Design review of the part built by this model. Coordinates are the model's own, in mm. Give positions to 0.01 mm unless a question says otherwise; leave off trailing zeros.
```python
from build123d import *

# Parameters (mm, degrees)
SKETCH3_R          = 5
SKETCH6_R          = 5
SKETCH7_R          = 7.5
CUT_EXTRUDE1_DEPTH = 123.474487302


with BuildPart() as part:
    # Sketch1 → Loft1 section 0
    with BuildSketch(Plane(origin=(0, 0, 0), x_dir=(0, 0, -1), z_dir=(1, 0, 0))):
        with BuildLine():
            Line((40, 40), (-40, 40))
            Line((-40, 40), (-40, -40))
            Line((-40, -40), (40, -40))
            Line((40, -40), (40, 40))
        make_face()
    # Sketch2 → Loft1 section 1
    with BuildSketch(Plane(origin=(-100, 0, 0), x_dir=(0, 0, -1), z_dir=(1, 0, 0))):
        with BuildLine():
            Line((50, 50), (-50, 50))
            Line((-50, 50), (-50, -50))
            Line((-50, -50), (50, -50))
            Line((50, -50), (50, 50))
        make_face()
    loft()

    # Cut-Sweep2: sweep along a path in Sketch4
    with BuildLine(Plane(origin=(0, 0, 0), x_dir=(1, 0, 0), z_dir=(0, 1, 0))) as cut_sweep2_path:
        Line((0, 15), (-100, 25))
    # Sketch3 → Cut-Sweep2 (sweep, cut)
    with BuildSketch(Plane(origin=(0, 0, 0), x_dir=(0, 0, -1), z_dir=(1, 0, 0))):
        with Locations((15, 0)):
            Circle(SKETCH3_R)
    cut_sweep2 = sweep(path=cut_sweep2_path.line, mode=Mode.SUBTRACT)

    # Cut-Sweep3: sweep along a path in Sketch5
    with BuildLine(Plane.XY) as cut_sweep3_path:
        Line((0, 15), (-100, 25))
    # Sketch6 → Cut-Sweep3 (sweep, cut)
    with BuildSketch(Plane(origin=(0, 0, 0), x_dir=(0, 0, -1), z_dir=(1, 0, 0))):
        with Locations((0, 15)):
            Circle(SKETCH6_R)
    cut_sweep3 = sweep(path=cut_sweep3_path.line, mode=Mode.SUBTRACT)

    # Mirror1: Cut-Sweep2 across plane
    add(cut_sweep2.mirror(Plane.XY), mode=Mode.SUBTRACT)

    # Mirror2: Cut-Sweep3 across plane
    add(cut_sweep3.mirror(Plane.ZX), mode=Mode.SUBTRACT)

    # Sketch7 → Cut-Extrude1 (cut, through all)
    with BuildSketch(Plane(origin=(0, 0, 0), x_dir=(0, 0, -1), z_dir=(1, 0, 0))):
        Circle(SKETCH7_R)
    extrude(amount=-CUT_EXTRUDE1_DEPTH, mode=Mode.SUBTRACT)


solid = part.part
```
1. Draft analysis for pull direction Z (two halves, no side actions). For faces 1 (the face through (-49.3, 0.33, 7.493)), 2 (the face through (-100, 13, 11)), state which applies: pulls with the +Z half, pulls with the -Z half, needs draft (parallel to the pull), parting line crosses it, or undercut.
Recorded:
face 1: undercut
face 2: needs draft
2. For line 1 along Y through (x, z) = (-68, 4.5); line 2 along Z through (x, y) = (-31.5, -1); line 3 along Y through (x, z) = (-47, 0), list the stretches that pass through material, from the lowest coordinate up.
Recorded:
line 1: y = -46.8 to -23.98, -19.62 to -6, 6 to 19.62, 23.98 to 46.8
line 2: z = -43.15 to -23.05, -13.25 to -7.43, 7.43 to 13.25, 23.05 to 43.15
line 3: y = -44.7 to -24.7, -14.7 to -7.5, 7.5 to 14.7, 24.7 to 44.7
3. For pin 1 (1.5 mm diameter, centred on x = -46, y = 11, fed in from +Z) (3 decimals); pin 2 (10 mm diameter, centred on x = -47, y = -27, fed in from -Z); pin 3 (10 mm diameter, centred on x = -88.5, z = -36.5, fed in from -Y), all flat-tipped, find the tip position at first contact; note any pin that passes through.
Recorded:
pin 1: stops at z = 44.675
pin 2: stops at z = -45.2
pin 3: stops at y = -49.35
4. Take a section at A-A (y = 0). State how many separate pieces and enclosed holes the cut face has, then the cut area to 3 significant figures.
Recorded:
separate pieces: 4
enclosed holes: 0
area: 5,500 mm2
